Here's how the part is built. I have some questions about the finished solid (model axes, mm). A direction names the side the tool comes from. Round coordinates to 2 decimals unless told otherwise and drop trailing zeros. Loops run counter-clockwise (first coordinate to the right, second up) from the corner with the lowest first, then second, coordinate; pieces in that order, holes last. Notation, with made-up numbers: M 7.25,64.5 L 24.25,64.5 A12 ccw 24.25,71.5 Z; hole C 9,29 d8. An arc over 180 degrees is marked long. Write each question's results on one line, items separated by ' | '. Start each with the question number.
```python
from build123d import *

# Parameters (mm, degrees)
SKETCH1_R           = 56.35625
SKETCH1_R_2         = 50.00625
BOSS_EXTRUDE1_DEPTH = 3.571875
HOLE1_D             = 3.175
HOLE1_DEPTH         = 12.7
HOLE1_CBORE_D       = 6.35
HOLE1_CBORE_DEPTH   = 3.175


with BuildPart() as part:
    # Sketch1 → Boss-Extrude1 (new body, symmetric)
    with BuildSketch(Plane.XY):
        Circle(SKETCH1_R)
        Circle(SKETCH1_R_2, mode=Mode.SUBTRACT)
    extrude(amount=BOSS_EXTRUDE1_DEPTH, both=True)

    # Hole1
    with Locations(Plane.YZ.offset(56.35625)):
        with Locations((0, 0)):
            hole1 = CounterBoreHole(HOLE1_D / 2, HOLE1_CBORE_D / 2, HOLE1_CBORE_DEPTH, depth=HOLE1_DEPTH)

    # Mirror1: Hole1 across plane
    add(hole1.mirror(Plane(origin=(0, 0, 0), x_dir=(0, 0, 1), z_dir=(1, 0, 0))), mode=Mode.SUBTRACT)


solid = part.part
```
Item 1: If we section it at A-A on y = 0: Count the separate pieces of the cut face and the enclosed holes in it, and give its area (3 significant figures).
Item 2: I'm going to push flat-ended pins straight in: pin 1 (1.9 mm diameter, centred on y = 1.5, z = 1, fed in from -X); pin 2 (2.5 mm diameter, centred on y = 0, z = 0, fed in from -X); pin 3 (4 mm diameter, centred on y = 0, z = 0, fed in from +X); pin 4 (1 mm diameter, centred on y = 26, z = -0.5, fed in from -X). Where does each tip first touch, or does it pass through?
Item 3: If we mould it in two halves opening along Y, with no side actions, what happens to faces 1 (the face through (53.754, 16.928, 0.05)), 2 (the face through (-21, -46, -3.572)), 3 (the face through (-10.84, -48.817, -0.05))? For each: released by +Y, released by -Y, zero draft, split by the parting line, or undercut.
Item 4: If we section it at B-B on x = 0: Please give me the cut outline in (y, z).
Item 5: If we section it at D-D on y = 31: Please give me the cut outline in (x, z).
Item 6: I need wall thicknesses on L1, parallel to Y at x = 0.5, z = 3.25; L2, parallel to X at y = 0, z = -2; L3, parallel to X at y = 46.5, z = -0.75. Which ranges of each line are inside material? Lowest first, please.
Item 7: Which directions (+Z, -Z, +X, -X, +Y, -Y) give clear straight access to the entire face, cutting with the end or side of a thin tool? Please do faces 4 (the face through (-54.79, -0.69, -3.1)), 5 (the face through (54.79, -0.69, -3.1)), 6 (the face through (-21, -46, 3.572)).
Numbers:
1) separate pieces: 4 | enclosed holes: 0 | area: 30.2 mm²
2) pin 1: x = -53.18 | pin 2: through | pin 3: x = 53.18 | pin 4: x = -50.26
3) face 1: split by the parting line | face 2: zero draft | face 3: undercut
4) outline: M -56.36,-3.57 L -50.01,-3.57 L -50.01,3.57 L -56.36,3.57 Z; M 50.01,-3.57 L 56.36,-3.57 L 56.36,3.57 L 50.01,3.57 Z
5) outline: M -47.06,-3.57 L -39.24,-3.57 L -39.24,3.57 L -47.06,3.57 Z; M 39.24,-3.57 L 47.06,-3.57 L 47.06,3.57 L 39.24,3.57 Z
6) L1: -56.35 to -50, 50 to 56.35 | L2: -53.18 to -50.01, 50.01 to 53.18 | L3: -31.84 to -18.39, 18.39 to 31.84
7) face 4: -X | face 5: +X | face 6: +Z, +X, -X, +Y, -Y
